from build123d import *

# Parameters (mm, degrees)
ESQUISSE1_W      = 95
ESQUISSE1_H      = 38
EXTRUSION1_DEPTH = 10
ESQUISSE3_R      = 12
EXTRUSION3_DEPTH = 8
ESQUISSE4_W      = 5.8
ESQUISSE4_H      = 38
EXTRUSION4_DEPTH = 2


with BuildPart() as part:
    # Esquisse1 → Extrusion1 (new body)
    with BuildSketch(Plane.XY):
        with Locations((47.5, -19)):
            Rectangle(ESQUISSE1_W, ESQUISSE1_H)
        with BuildLine():
            ThreePointArc((46.263573917, -10.349264706), (40.788303121, -14.125), (40.256055836, -20.754591249))
            ThreePointArc((40.256055836, -20.754591249), (38.839745962, -23), (41.492481919, -22.896144045))
            ThreePointArc((41.492481919, -22.896144045), (47.5, -25.75), (53.507518081, -22.896144045))
            ThreePointArc((53.507518081, -22.896144045), (56.160254038, -23), (54.743944164, -20.754591249))
            ThreePointArc((54.743944164, -20.754591249), (54.211696879, -14.125), (48.736426083, -10.349264706))
            ThreePointArc((48.736426083, -10.349264706), (47.5, -8), (46.263573917, -10.349264706))
        make_face(mode=Mode.SUBTRACT)
    extrude(amount=EXTRUSION1_DEPTH)

    # Esquisse3 → Extrusion3 (cut)
    with BuildSketch(Plane.XY.offset(10)):
        with Locations((47.5, -18)):
            Circle(ESQUISSE3_R)
    extrude(amount=-EXTRUSION3_DEPTH, mode=Mode.SUBTRACT)

    # Esquisse4 → Extrusion4 (cut)
    with BuildSketch(Plane.XY.offset(10)):
        with Locations((8, -19)):
            Rectangle(ESQUISSE4_W, ESQUISSE4_H)
        with Locations((87, -19)):
            Rectangle(ESQUISSE4_W, ESQUISSE4_H)
    extrude(amount=-EXTRUSION4_DEPTH, mode=Mode.SUBTRACT)


solid = part.part
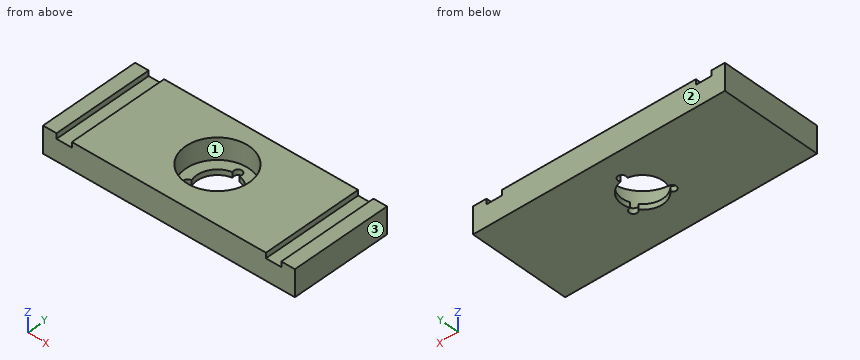
Work out the finished part from the listing and answer in its coordinate system (mm). Face numbers are marked on the shaded views. Give positions to 0.01 mm unless a question says otherwise; leave off trailing zeros. Order: outer loops, then holes, each group sorted by start corner. A loop starts at its lowest first (then second) coordinate and runs counter-clockwise, first axis right, second up. Notation, with made-up numbers: M -1.5,-4.75 L 38.5,-4.75 A20 cw 38.5,-0.75 Z; hole C 75,-22.5 d2. An arc over 180 degrees is marked long. Return JSON: item names as keys, results as strings.
Q1. Find the intervals of material crossed by line 1 along Y through (x, z) = (47.5, 1.45); line 2 along X through (y, z) = (-22.25, 1.15); line 3 along Y through (x, z) = (47.5, 5), in increasing order. Write a range as [from, to].
Answer below:
{"line 1": "y = [-38, -25.75], [-8, 0]", "line 2": "x = [0, 38.64], [56.36, 95]", "line 3": "y = [-38, -30], [-6, 0]"}
Q2. Find section B-B, the plane y = -18. Write down the section's boundary in (x, z).
Answer below:
{"outline": "M 0,0 L 39.75,0 L 39.75,2 L 35.5,2 L 35.5,10 L 10.9,10 L 10.9,8 L 5.1,8 L 5.1,10 L 0,10 Z; M 55.25,0 L 95,0 L 95,10 L 89.9,10 L 89.9,8 L 84.1,8 L 84.1,10 L 59.5,10 L 59.5,2 L 55.25,2 Z"}
Q3. Find section C-C, the plane z = 3.5. Write down the section's boundary in (x, y), and give its area (3 significant figures).
Answer below:
{"outline": "M 0,-38 L 95,-38 L 95,0 L 0,0 Z; hole C 47.5,-18 d24", "area": "3,160 mm^2"}
Q4. The mould has two halves that part along Y. Classify the marked faces 1, 2 and 3: pulls with the +Y half, pulls with the -Y half, needs draft (parallel to the pull), parting line crosses it, or undercut.
Answer below:
{"face 1": "undercut", "face 2": "pulls with the +Y half", "face 3": "needs draft"}
Q5. Find section A-A, the plane x = 47.5. Write down the section's boundary in (y, z), and give its area (4 significant figures).
Answer below:
{"outline": "M -38,0 L -25.75,0 L -25.75,2 L -30,2 L -30,10 L -38,10 Z; M -8,0 L 0,0 L 0,10 L -6,10 L -6,2 L -8,2 Z", "area": "152.5 mm^2"}
Q6. Find section D-D, the plane y = -9.5. Write down the section's boundary in (x, z).
Answer below:
{"outline": "M 0,0 L 46,0 L 46,2 L 39.03,2 L 39.03,10 L 10.9,10 L 10.9,8 L 5.1,8 L 5.1,10 L 0,10 Z; M 49,0 L 95,0 L 95,10 L 89.9,10 L 89.9,8 L 84.1,8 L 84.1,10 L 55.97,10 L 55.97,2 L 49,2 Z"}
Q7. Each of these flat-tipped pins is pushed along its axis until it touches: pin 1 (1.7 mm diameter, centred on x = 86.5, y = -23, fed in from +Z); pin 2 (2.5 mm diameter, centred on x = 47.5, y = -9.5, fed in from +Z); pin 3 (12 mm diameter, centred on x = 51, y = -19, fed in from +Z). Where does it stop, or does it pass through?
Answer below:
{"pin 1": "stops at z = 8", "pin 2": "passes through", "pin 3": "stops at z = 2"}
